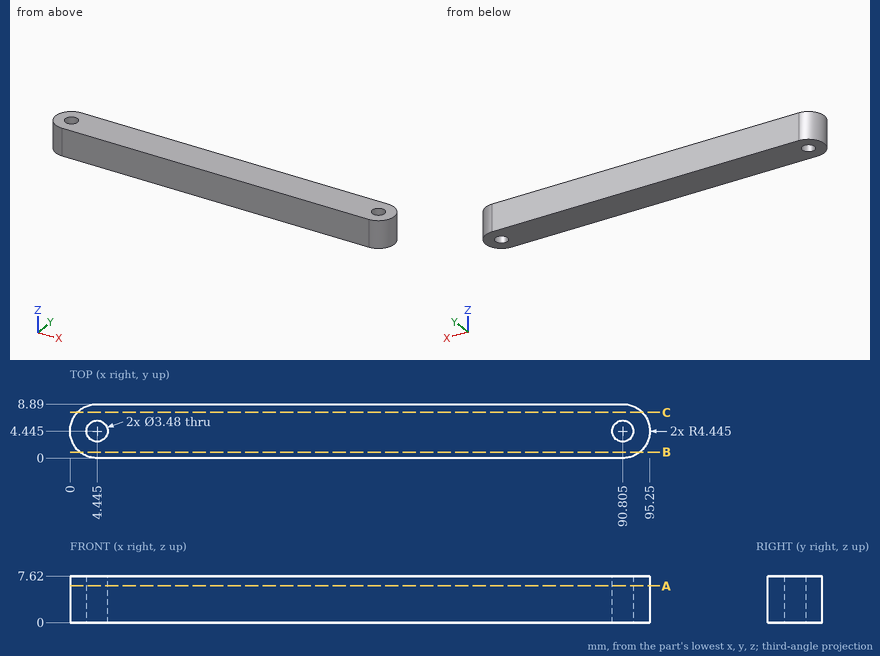
Here's the drawing with two shaded views (mm, measured from the low corner). I have some questions. Give positions to 0.01 mm unless a question says otherwise; leave off trailing zeros. Loops run counter-clockwise (first coordinate to the right, second up) from the corner with the lowest first, then second, coordinate; pieces in that order, holes last. Notation, with made-up numbers: M -32.5,89 L 4.5,89 A20 ccw 4.5,99 Z; hole C -7.75,68 d8. An arc over 180 degrees is marked long. One line per item, written item: value.
1) Imagine slicing it at A-A on z = 6. Write out the boundary of the cut face in (x, y) (1 decimal), and give its area (3 significant figures).
Geometry check:
outline: M 4.4,0 L 90.8,0 A4.4 ccw 90.8,8.9 L 4.4,8.9 A4.4 ccw Z; hole C 4.4,4.4 d3.5; hole C 90.8,4.4 d3.5
area: 811 mm²
2) I'm going to push a flat-ended pin straight in: pin 1 (1.5 mm diameter, centred on y = 8, z = 5.5, fed in from -X). Where does the tip first touch, or does it pass through?
Geometry check:
pin 1: stops at x = 1
3) Please list where these lines run through material, in increasing order: line 1 (X direction, y = 4.75, z = 1); line 2 (Y direction, x = 6, z = 5.75) (1 decimal); line 3 (X direction, y = 5.5, z = 3.75).
Geometry check:
line 1: x = 0.01 to 2.73, 6.16 to 89.09, 92.52 to 95.24
line 2: y = 0 to 3.7, 5.2 to 8.9
line 3: x = 0.13 to 3.06, 5.83 to 89.42, 92.19 to 95.12
4) Imagine slicing it at C-C on y = 7.5. Write out the boundary of the cut face in (x, z), and give its area (3 significant figures).
Geometry check:
outline: M 1.22,0 L 94.03,0 L 94.03,7.62 L 1.22,7.62 Z
area: 707 mm²
5) Imagine slicing it at B-B on y = 1. Write out the boundary of the cut face in (x, z).
Geometry check:
outline: M 1.64,0 L 93.61,0 L 93.61,7.62 L 1.64,7.62 Z
